```python
from build123d import *

# Parameters (mm, degrees)
BOSS_EXTRUDE7_DEPTH = 20
SKETCH12_R          = 31.514643475
BOSS_EXTRUDE8_DEPTH = 100


with BuildPart() as part:
    # Sketch1 → Boss-Extrude7 (new body)
    with BuildSketch(Plane.XY):
        Polygon((-74.036406968, -41.544157833), (-74.036406968, -29.88599594), (-265.556443783, -29.88599594), (-206.925428257, -38.639637749), (-121.846026988, -38.639637749), (-116.925428257, -41.544157833), align=None)
        Polygon((-74.036406968, -29.88599594), (-74.036406968, -18.227834048), (-116.925428257, -18.227834048), (-121.846026988, -21.132354132), (-206.925428257, -21.132354132), (-265.556443783, -29.88599594), align=None)
        Polygon((-60, -59.771991881), (-60, -29.88599594), (-74.036406968, -29.88599594), (-74.036406968, -41.544157833), (-74.036406968, -51.486612768), align=None)
        Polygon((-60, -29.88599594), (-60, 0), (-74.036406968, -8.285379113), (-74.036406968, -18.227834048), (-74.036406968, -29.88599594), align=None)
    extrude(amount=BOSS_EXTRUDE7_DEPTH)

    # Sketch12 → Boss-Extrude8 (add)
    with BuildSketch(Plane(origin=(-60, 0, 0), x_dir=(0, 0, -1), z_dir=(1, 0, 0))):
        with Locations(Location((-10, -29.88599594, 0), (0, 0, 251.499507524))):
            Circle(SKETCH12_R)
    extrude(amount=BOSS_EXTRUDE8_DEPTH)


solid = part.part
```
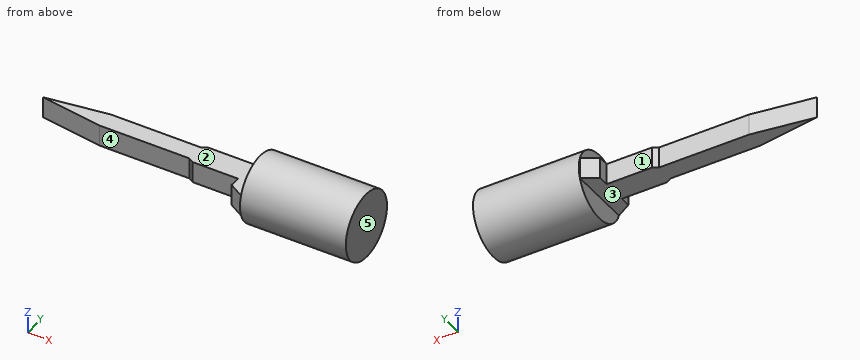
The model under review builds one solid part; all positions refer to its coordinate system, in mm. Face numbers are marked on the shaded views. A direction names the side the tool comes from. Give positions to 0.01 mm unless a question says otherwise; leave off trailing zeros. Write each loop counter-clockwise with the first axis right and the second up, starting at its lowest first coordinate (ties: lowest second). Pieces come first, ordered by that corner, then holes. Notation, with made-up numbers: M 58.5,-3 L 97.5,-3 A11 ccw 97.5,12 Z; hole C -18.75,18 d9. An arc over 180 degrees is marked long. Write each question's results on one line, items separated by ' | '. Start each with the question number.
1. Insertion check: pin 1 Ø6 at (x, z) = (-166, 8.5) entering from -Y; pin 2 Ø6.5 at (y, z) = (-23.5, 30) entering from -X; pin 3 Ø8 at (y, z) = (-11, 5.5) entering from -X. Each pin has a flat end and moves straight along its axis. Give the tip position at first contact, or say it passes through.
2. We need section D-D (x = -104). Write out the cut boundary in (y, z), and give its area (3 significant figures).
3. We need section B-B (x = -138). Write out the cut boundary in (y, z), and give its area (3 significant figures).
4. We need section A-A (z = 10). Write out the cut boundary in (x, y), and give its area (3 significant figures).
5. For probe 1 along X at (y, z) = (-50.5, -1); probe 2 along Y at (x, z) = (-126, 17.5); probe 3 along Z at (x, y) = (-67.5, -39), list the stretches that pass through material, from the lowest coordinate up. Write a range as [from, to].
6. For the marked faces 1, 2, 3, 4 and 5, list the 3-axis set-ups (+Z, -Z, +X, -X, +Y, -Y) from which the entire face can be reached by the end or side of a thin tool; tool diameter is ignored.
7. We need section C-C (y = -4). Write out the cut boundary in (x, z), and give its area (3 significant figures).
Results found:
1) pin 1: stops at y = -38.64 | pin 2: stops at x = -60 | pin 3: stops at x = -74.04
2) outline: M -41.54,0 L -18.23,0 L -18.23,20 L -41.54,20 Z | area: 466 mm^2
3) outline: M -38.64,0 L -21.13,0 L -21.13,20 L -38.64,20 Z | area: 350 mm^2
4) outline: M -265.56,-29.89 L -206.93,-38.64 L -121.85,-38.64 L -116.93,-41.54 L -74.04,-41.54 L -74.04,-51.49 L -60,-59.77 L -60,-61.4 L 40,-61.4 L 40,1.63 L -60,1.63 L -60,0 L -74.04,-8.29 L -74.04,-18.23 L -116.93,-18.23 L -121.85,-21.13 L -206.93,-21.13 Z | area: 10,100 mm^2
5) probe 1: x = [-60, 40] | probe 2: y = [-38.64, -21.13] | probe 3: z = [0, 20]
6) face 1: +Z, -Z, -X, +Y | face 2: +Z, -X, +Y, -Y | face 3: -Z, -X, +Y, -Y | face 4: +Z, -Z, -X, -Y | face 5: +Z, -Z, +X, +Y, -Y
7) outline: M -66.78,0 L -60,0 L -60,-7.97 L 40,-7.97 L 40,27.97 L -60,27.97 L -60,20 L -66.78,20 Z | area: 3,730 mm^2
